Input: part model. Units: mm. Frame: model coordinates. A direction names the side the tool comes from. Give positions to 0.01 mm unless a question says otherwise; leave off trailing zeros. Write each loop counter-clockwise with the first axis right and the second up, starting at its lowest first coordinate (ties: lowest second). Pieces come first, ordered by that corner, then holes. Notation, with made-up numbers: (72, -30) - (104, -30) arc R33 cw to (104, -2) - close; hole circle Ø7 at (79.25, 22). An arc over 180 degrees is marked (long way). Use a Markdown table: item, result. Add a question column.
1. Section query B-B, the plane x = -2.25. Return loops of the section in (y, z).
2. Section query C-C, the plane z = 3. Return loops of the section in (x, y), plus the area to 3 significant figures.
3. Material intervals for probe 1 along Z at (x, y) = (1.7, 0); probe 2 along Z at (x, y) = (2, 2.75); probe 3 along Y at (x, z) = (1.6, 3), sorted ascending.
4. Section query A-A, the plane y = 0. Return loops of the section in (x, z).
5. Pin query (flat end, axial travel): pin 1 (3 mm diameter, centred on y = -1, z = 14.5, fed in from +X); pin 2 (1.5 mm diameter, centred on y = 2, z = 4.5, fed in from +X); pin 3 (1 mm diameter, centred on x = -1, z = 18.5, fed in from +Y); pin 4 (1 mm diameter, centred on x = -2.5, y = 1, fed in from -Z). Return the tip coordinate at first contact, or that it passes through.
6. Section query D-D, the plane z = 7.5. Return loops of the section in (x, y).
7. Mould query, pull axis X, two halves, no side actions, for faces 1 (the cylindrical face through (-0.867, -3.905, 21.479)), 2 (the flat face through (0, 0, 8)), 3 (the flat face through (1, 3, 20)). Classes: released by +X, released by -X, zero draft, split by the parting line, or undercut.
8. Set-up query: faces 4 (the cylindrical face through (-2, 2, 3)), 5 (the cylindrical face through (2.86, 0.9, 9.86)), 6 (the flat face through (-1, 1, 5)). Return all of +Z, -Z, +X, -X, +Y, -Y with unobstructed straight access to the full face (end or side cutting, diameter ignored); none if empty.
```python
from build123d import *

# Parameters (mm, degrees)
SKETCH_1_R          = 3
EXTRUDE_1_DEPTH     = 20
SKETCH_2_R          = 4
EXTRUDE_2_DEPTH     = 3
SKETCH_4_W          = 2
SKETCH_4_H          = 6.835299346
CUT_EXTRUDE_1_DEPTH = 8
SKETCH_5_R          = 2
CUT_EXTRUDE_2_DEPTH = 4


with BuildPart() as part:
    # 草图1 → 凸台-拉伸1 (new body)
    with BuildSketch(Plane.XY):
        Circle(SKETCH_1_R)
    extrude(amount=EXTRUDE_1_DEPTH)

    # 草图2 → 凸台-拉伸2 (add)
    with BuildSketch(Plane.XY.offset(20)):
        Circle(SKETCH_2_R)
    extrude(amount=EXTRUDE_2_DEPTH)

    # 草图4 → 切除-拉伸1 (cut)
    with BuildSketch(Plane(origin=(0, 0, 0), x_dir=(-1, 0, 0), z_dir=(0, 0, -1))):
        Rectangle(SKETCH_4_W, SKETCH_4_H)
    extrude(amount=-CUT_EXTRUDE_1_DEPTH, mode=Mode.SUBTRACT)

    # 草图5 → 切除-拉伸2 (cut, symmetric)
    with BuildSketch(Plane(origin=(0, 0, 0), x_dir=(0, 0, -1), z_dir=(1, 0, 0))):
        with Locations((-3, 0)):
            Circle(SKETCH_5_R)
    extrude(amount=CUT_EXTRUDE_2_DEPTH, both=True, mode=Mode.SUBTRACT)


solid = part.part
```
Result sheet:
| question | item | result |
|---|---|---|
| 1 | outline | (-3.31, 20) - (-1.98, 20) - (-1.98, 3.25) arc R2 cw to (1.98, 3.25) - (1.98, 20) - (3.31, 20) - (3.31, 23) - (-3.31, 23) - close; (-1.98, 0) - (1.98, 0) - (1.98, 2.75) arc R2 cw to (-1.98, 2.75) - close |
| 2 | outline | (-2.24, -2) arc R3 ccw to (-1, -2.83) - (-1, -2) - close; (-2.24, 2) - (-1, 2) - (-1, 2.83) arc R3 ccw to start; (1, -2.83) arc R3 ccw to (2.24, -2) - (1, -2) - close; (1, 2) - (2.24, 2) arc R3 ccw to (1, 2.83) - close |
| 2 | area | 2.42 mm² |
| 3 | probe 1 | z = 0 to 1, 5 to 23 |
| 3 | probe 2 | z = 20 to 23 |
| 3 | probe 3 | y = -2.54 to -2, 2 to 2.54 |
| 4 | outline | (-4, 20) - (-3, 20) - (-3, 5) - (-1, 5) - (-1, 8) - (1, 8) - (1, 5) - (3, 5) - (3, 20) - (4, 20) - (4, 23) - (-4, 23) - close; (-3, 0) - (-1, 0) - (-1, 1) - (-3, 1) - close; (1, 0) - (3, 0) - (3, 1) - (1, 1) - close |
| 5 | pin 1 | stops at x = 3 |
| 5 | pin 2 | stops at x = 2.73 |
| 5 | pin 3 | stops at y = 2.96 |
| 5 | pin 4 | stops at z = 0 |
| 6 | outline | (-1, -2.83) - (-1, 2.83) arc R3 ccw to start; (1, -2.83) arc R3 ccw to (1, 2.83) - close |
| 7 | face 1 | split by the parting line |
| 7 | face 2 | undercut |
| 7 | face 3 | zero draft |
| 8 | face 4 | +X, -X |
| 8 | face 5 | -Z |
| 8 | face 6 | -Z, +Y, -Y |
